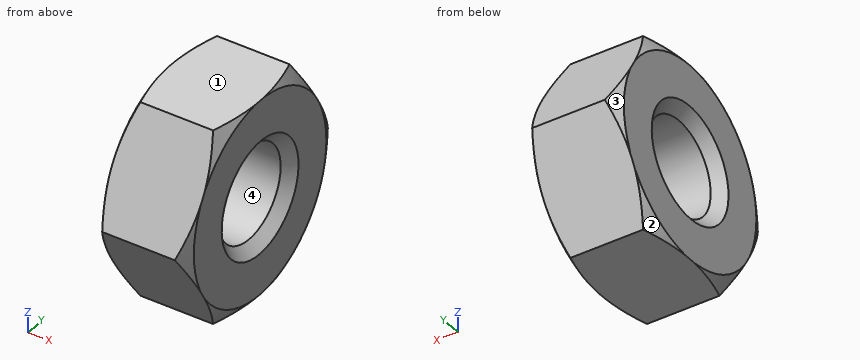
from build123d import *

# Parameters (mm, degrees)
SKETCH1_R           = 1.65
BOSS_EXTRUDE1_DEPTH = 1.6
CHAMFER1_SIZE       = 0.379


with BuildPart() as part:
    # Sketch1 → Boss-Extrude1 (new, symmetric)
    with BuildSketch(Plane(origin=(0, 0, 0), x_dir=(0, 0, -1), z_dir=(1, 0, 0))):
        Polygon((3.5, 2.020725942), (3.5, -2.020725942), (0, -4.041451884), (-3.5, -2.020725942), (-3.5, 2.020725942), (0, 4.041451884), align=None)
        Circle(SKETCH1_R, mode=Mode.SUBTRACT)
    extrude(amount=BOSS_EXTRUDE1_DEPTH, both=True)

    # Sketch4 → Cut-Revolve1 (revolve, cut)
    with BuildSketch(Plane.XY):
        Polygon((-1.6, 3.5), (-1.6, 5.227530151), (-0.602610002, 5.227530151), align=None)
    cut_revolve1 = revolve(axis=Axis((-2.7190736, 0, 0), (1, 0, 0)), mode=Mode.SUBTRACT)

    # Mirror1: Cut-Revolve1 across plane
    add(cut_revolve1.mirror(Plane(origin=(0, 0, 0), x_dir=(0, 0, 1), z_dir=(1, 0, 0))), mode=Mode.SUBTRACT)

    # Chamfer1
    chamfer1_edges = [part.edges().sort_by_distance(p)[0] for p in [
        (-1.6, 0, 1.65),
        (1.6, 0, 1.65),
    ]]
    chamfer(chamfer1_edges, length=CHAMFER1_SIZE)


solid = part.part
Could you check a few things on this model? Use its own coordinates, in mm. Face numbers are marked on the shaded views. Give positions to 0.01 mm unless a question says otherwise; leave off trailing zeros. Order: outer loops, then holes, each group sorted by start corner. A loop starts at its lowest first (then second) coordinate and runs counter-clockwise, first axis right, second up.
1. For pin 1 (3 mm diameter, centred on y = 0, z = 0, fed in from +X), with a flat end and sliding along its axis, tell me the tip position at first contact or that it passes through.
Answers below:
pin 1: passes through
2. Thinking about a two-plate mould opening in Z: for the marked faces 1, 2, 3 and 4, which applies, +Z half, -Z half, draft (parallel to the pull), parting line (faces both ways), or undercut?
Answers below:
face 1: +Z half
face 2: -Z half
face 3: parting line
face 4: undercut
3. Suppose I cut it at A-A (x = 0.1). Write out the boundary of the cut face in (y, z), plus the area to 3 significant figures.
Answers below:
outline: (-4.04, 0) - (-2.02, -3.5) - (2.02, -3.5) - (4.04, 0) - (2.02, 3.5) - (-2.02, 3.5) - close; hole circle Ø3.3 at (0, 0)
area: 33.9 mm2
4. I need wall thicknesses on L1, parallel to Z at x = 0.1, y = -0.5; L2, parallel to Z at x = 1.3, y = -1; L3, parallel to Y at x = 1.15, z = 1.25. Which ranges of each line are inside material? Lowest first, please.
Answers below:
L1: z = -3.5 to -1.57, 1.57 to 3.5
L2: z = -3.5 to -1.41, 1.41 to 3.5
L3: y = -3.32 to -1.08, 1.08 to 3.32
